```python
from build123d import *

# Parameters (mm, degrees)
SKETCH_1_W      = 45
SKETCH_1_H      = 45
EXTRUDE_1_DEPTH = 2
FILLET_1_R      = 15
SKETCH_2_W      = 40.8
SKETCH_2_H      = 40.8
EXTRUDE_2_DEPTH = 2
FILLET_2_R      = 13
SHELL_1_T       = -2


with BuildPart() as part:
    # 스케치1 → 보스-돌출1 (new body)
    with BuildSketch(Plane.XY):
        with Locations((11.279766248, -4.096820809)):
            Rectangle(SKETCH_1_W, SKETCH_1_H)
    extrude(amount=EXTRUDE_1_DEPTH)

    # 필렛1
    fillet_1_edges = [part.edges().sort_by_distance(p)[0] for p in [
        (-11.220233752, 18.403179191, 1),
        (33.779766248, 18.403179191, 1),
        (33.779766248, -26.596820809, 1),
        (-11.220233752, -26.596820809, 1),
    ]]
    fillet(fillet_1_edges, radius=FILLET_1_R)

    # 스케치2 → 보스-돌출2 (add)
    with BuildSketch(Plane.XY.offset(2)):
        with Locations((11.279766248, -4.096820809)):
            Rectangle(SKETCH_2_W, SKETCH_2_H)
    extrude(amount=EXTRUDE_2_DEPTH)

    # 필렛2
    # the kernel refuses this fillet: 13 mm, written as the material it takes off along each edge
    with BuildSketch(Plane(origin=(31.679766248, -24.496820809, 2), x_dir=(0, 1, 0), z_dir=(0, 0, 1)), Plane(origin=(31.679766248, 16.303179191, 2), x_dir=(-1, 0, 0), z_dir=(0, 0, 1))) as fillet_2_piece_1:
        with BuildLine():
            CenterArc((FILLET_2_R, FILLET_2_R), FILLET_2_R, 180, 90)
            Line((0, FILLET_2_R), (0, 0))
            Line((0, 0), (FILLET_2_R, 0))
        make_face()
    extrude(amount=34.5, mode=Mode.SUBTRACT)
    with BuildSketch(Plane(origin=(-9.120233752, 16.303179191, 2), x_dir=(1, 0, 0), z_dir=(0, 0, 1)), Plane(origin=(-9.120233752, -24.496820809, 2), x_dir=(0, 1, 0), z_dir=(0, 0, 1))) as fillet_2_piece_2:
        with BuildLine():
            CenterArc((FILLET_2_R, -FILLET_2_R), FILLET_2_R, 90, 90)
            Line((0, -FILLET_2_R), (0, 0))
            Line((0, 0), (FILLET_2_R, 0))
        make_face()
    extrude(amount=34.5, mode=Mode.SUBTRACT)

    # 쉘1
    shell_1_openings = [part.faces().sort_by_distance(p)[0] for p in [
        (11.279766248, -4.096820809, 4),
    ]]
    offset(amount=SHELL_1_T, openings=shell_1_openings, kind=Kind.INTERSECTION)


solid = part.part
```
Geometry: final body of the model. Coordinates: model frame, mm. A direction names the side the tool comes from. Give positions to 0.01 mm unless a question says otherwise; leave off trailing zeros. Order: outer loops, then holes, each group sorted by start corner. A loop starts at its lowest first (then second) coordinate and runs counter-clockwise, first axis right, second up. Notation, with made-up numbers: (53, 48.5) -> (109, 48.5) arc R24 ccw to (109, 69.5) -> close; hole circle Ø1 at (-25, 40.5). An arc over 180 degrees is marked (long way). Write each question's results on one line, items separated by ' | '. Start each with the question number.
1) Section D-D (x = -8). Return loops of the section in (y, z), then the cut area to 3 significant figures.
2) Section A-A (z = 2.9). Return loops of the section in (x, y).
3) First-contact query: pin 1 (1.5 mm diameter, centred on y = -19.5, z = 1.5, fed in from -X); pin 2 (0.6 mm diameter, centred on x = 14, z = 3.5, fed in from -Y); pin 3 (0.6 mm diameter, centred on y = -3.5, z = 2.5, fed in from +X). Flat tips, straight axial feed; report the tip coordinate or a pass-through.
4) Section B-B (x = 23). Return loops of the section in (y, z).
5) Set-up query: faces 5 (the flat face through (11, -22.497, 3)), 6 (the flat face through (11, 16.303, 3)), 7 (the cylindrical face through (27.973, 12.394, 2.986)), 8 (the flat face through (-9.12, -4, 3)). Return all of +Z, -Z, +X, -X, +Y, -Y with unobstructed straight access to the full face (end or side cutting, diameter ignored); none if empty.
6) Section C-C (y = -9). Return loops of the section in (x, z), then the cut area to 3 significant figures.
7) Draft query along X for faces 1 (the flat face through (-7.12, -4, 3)), 2 (the flat face through (-11.22, -4, 1)), 3 (the flat face through (11, 18.403, 1)), 4 (the flat face through (31.68, -4, 3)). Return one class per face: pulls with the +X half, pulls with the -X half, needs draft (parallel to the pull), parting line crosses it, or undercut.
8) Line query: line 1 (Y direction, x = 8, z = 3.4); line 2 (X direction, y = 1, z = 3.45); line 3 (Y direction, x = -1, z = 2.4). Output: solid intervals per line, ascending. Write a range as from..to.
Calculated:
1) outline: (-20.88, 0) -> (12.69, 0) -> (12.69, 2) -> (8.58, 2) -> (8.58, 4) -> (-16.78, 4) -> (-16.78, 2) -> (-20.88, 2) -> close | area: 118 mm2
2) outline: (-9.12, -11.5) arc R13 ccw to (3.88, -24.5) -> (18.68, -24.5) arc R13 ccw to (31.68, -11.5) -> (31.68, 3.3) arc R13 ccw to (18.68, 16.3) -> (3.88, 16.3) arc R13 ccw to (-9.12, 3.3) -> close; hole (-7.12, -11.5) arc R11 ccw to (3.88, -22.5) -> (18.68, -22.5) arc R11 ccw to (29.68, -11.5) -> (29.68, 3.3) arc R11 ccw to (18.68, 14.3) -> (3.88, 14.3) arc R11 ccw to (-7.12, 3.3) -> close
3) pin 1: x = -9.4 | pin 2: y = -24.5 | pin 3: x = 31.68
4) outline: (-25.99, 0) -> (17.8, 0) -> (17.8, 2) -> (15.56, 2) -> (15.56, 4) -> (13.42, 4) -> (13.42, 2) -> (-21.61, 2) -> (-21.61, 4) -> (-23.76, 4) -> (-23.76, 2) -> (-25.99, 2) -> close
5) face 5: +Z | face 6: +Z, +X, -X, +Y | face 7: +Z, +X, +Y | face 8: +Z, -X, +Y, -Y
6) outline: (-11.22, 0) -> (33.78, 0) -> (33.78, 2) -> (31.68, 2) -> (31.68, 4) -> (29.68, 4) -> (29.68, 2) -> (-7.12, 2) -> (-7.12, 4) -> (-9.12, 4) -> (-9.12, 2) -> (-11.22, 2) -> close | area: 98.0 mm2
7) face 1: undercut | face 2: pulls with the -X half | face 3: needs draft | face 4: pulls with the +X half
8) line 1: -24.5..-22.5, 14.3..16.3 | line 2: -9.12..-7.12, 29.68..31.68 | line 3: -23.55..-21.36, 13.16..15.35
